Autodesk Inventor part; units mm, degrees
ref_plane "YZ Plane" through (0, 0, 0) normal (1, 0, 0) x (0, 1, 0)
ref_plane "XZ Plane" through (0, 0, 0) normal (0, 1, 0) x (-1, 0, 0)
ref_plane "XY Plane" through (0, 0, 0) normal (0, 0, 1) x (1, 0, 0)
sketch "card+border" plane through (0, 0, 0) normal (0, 0, 1) x (1, 0, 0)
  line L0 (-59.3579, 68.5808) -> (-59.3579, 10.0008)
  line L1 (-59.3579, 10.0008) -> (14.2921, 10.0008)
  line L2 (14.2921, 10.0008) -> (14.2921, 68.5808)
  line L3 (14.2921, 68.5808) -> (-59.3579, 68.5808)
  circle A0 centre (11.6671, 65.9558) radius 1.575
  circle A1 centre (11.6671, 12.6258) radius 1.575
  circle A2 centre (-56.7329, 65.9558) radius 1.575
  circle A3 centre (-56.7329, 12.6258) radius 1.575
  line L4 (-61.3579, 70.5808) -> (-61.3579, 8.0008)
  line L5 (-61.3579, 8.0008) -> (16.2921, 8.0008)
  line L6 (16.2921, 8.0008) -> (16.2921, 70.5808)
  line L7 (16.2921, 70.5808) -> (-61.3579, 70.5808)
  line L8 (-58.3579, 67.5808) -> (13.2921, 67.5808)
  line L9 (13.2921, 67.5808) -> (13.2921, 11.0008)
  line L10 (13.2921, 11.0008) -> (-58.3579, 11.0008)
  line L11 (-58.3579, 11.0008) -> (-58.3579, 67.5808)
  circle A4 centre (-56.7329, 65.9558) radius 3
  circle A5 centre (11.6671, 65.9558) radius 3
  circle A6 centre (11.6671, 12.6258) radius 3
  circle A7 centre (-56.7329, 12.6258) radius 3
  point P0 (0, 0)
  point P1 (-54.2111, 67.5808)
  point P2 (9.1454, 67.5808)
  point P3 (13.2921, 63.434)
  point P4 (13.2921, 15.1475)
  point P5 (9.1454, 11.0008)
  point P6 (-54.2111, 11.0008)
  point P7 (-58.3579, 15.1475)
  point P8 (-58.3579, 63.434)
  dimension "d1" = 58.58
  dimension "d2" = 73.65
  dimension "d4" = 2.625
  dimension "d5" = 3.15
  dimension "d31" = 2.625
  dimension "d32" = 2.625
  dimension "d33" = 2.625
  dimension "d34" = 3.15
  dimension "d35" = 2
  dimension "d36" = 3
  dimension "d37" = 3
  dimension "d38" = 3
  dimension "d39" = 3
  dimension "d40" = 6
  dimension "d41" = 6
  dimension "d42" = 6
  dimension "d43" = 6
extrude "Middle wall" add sketch "card+border" along normal blind 2 contours L3 A4 L0 | A4 L3 L8 L11 L0 | L0 A4 | A4 L3 | A4 L11 A7 L0 | L3 A5 L8 A4 | A7 L11 L10 L1 L0 | L0 A7 | L11 L8 A4 | A5 L3 | L3 A5 L2 L9 L8 | A7 L1 L0 | A7 L10 L11 | L3 L2 A5 | L8 L9 A5 | L1 A7 | A5 L2 | A5 L2 A6 L9 | A7 L10 A6 L1 | A6 L2 L1 L10 L9 | L9 L10 A6 | L1 A6 | A6 L2 | A6 L2 L1 | L7 L6 L5 L4
fillet "Skruehull suport" radius 2 8 edges at (9.1454, 67.5808, 1) (13.2921, 63.434, 1) (-58.3579, 63.434, 1) (-54.2111, 67.5808, 1) (-54.2111, 11.0008, 1) (-58.3579, 15.1475, 1) (13.2921, 15.1475, 1) (9.1454, 11.0008, 1)
fillet "Kantutjevning" radius 5 4 edges at (16.2921, 70.5808, 1) (-61.3579, 70.5808, 1) (-61.3579, 8.0008, 1) (16.2921, 8.0008, 1)
properties part number "Trippeldekker_Midtre plate"
CAD build for the part. Positions are in the model's coordinates, mm. A direction names the side the tool comes from. Coordinates: 2 decimals unless noted, no trailing zeros. Write each loop counter-clockwise with the first axis right and the second up, starting at its lowest first coordinate (ties: lowest second). Pieces come first, ordered by that corner, then holes. Notation, with made-up numbers: M 22,10 L 54,10 A21 ccw 54,45 Z; hole C 88.5,-16.75 d9. An arc over 180 degrees is marked long. Return JSON: item names as keys, results as strings.
Item 1: Slice it at C-C, the plane z = 1.25. Write the cut outline in (x, y) (3 decimals).
Findings below:
{"outline": "M -61.358,13.001 A5 ccw -56.358,8.001 L 11.292,8.001 A5 ccw 16.292,13.001 L 16.292,65.581 A5 ccw 11.292,70.581 L -56.358,70.581 A5 ccw -61.358,65.581 Z; hole M -58.358,17.612 A2 ccw -56.508,15.617 A3 cw -53.741,12.851 A2 ccw -51.747,11.001 L 6.681,11.001 A2 ccw 8.676,12.851 A3 cw 11.442,15.617 A2 ccw 13.292,17.612 L 13.292,60.97 A2 ccw 11.442,62.964 A3 cw 8.676,65.731 A2 ccw 6.681,67.581 L -51.747,67.581 A2 ccw -53.741,65.731 A3 cw -56.508,62.964 A2 ccw -58.358,60.97 Z; hole C -56.733,12.626 d3.15; hole C -56.733,65.956 d3.15; hole C 11.667,12.626 d3.15; hole C 11.667,65.956 d3.15"}
Item 2: Slice it at B-B, the plane y = 60. Write the cut outline in (x, z).
Findings below:
{"outline": "M -61.36,0 L -58.36,0 L -58.36,2 L -61.36,2 Z; M 13.29,0 L 16.29,0 L 16.29,2 L 13.29,2 Z"}
Item 3: Drop a flat-ended pin along its axis: pin 1 Ø3.5 at (x, y) = (11.67, 12.63) entering from -Z. Give the stop position or say it passes through.
Findings below:
{"pin 1": "stops at z = 0"}
Item 4: Which spindle directions (+Z, -Z, +X, -X, +Y, -Y) get a long thin tool onto all of the face, cutting with end or side? Do faces 4 (the cylindrical face through (-57.81, 62.345, 1.014)), 5 (the cylindrical face through (14.866, 69.077, 1.014)). Say none if no direction does.
Findings below:
{"face 4": "+Z, -Z", "face 5": "+Z, -Z, +X, +Y"}
Item 5: Probe line 1 (X direction, y = 33.5, z = 1); line 2 (Y direction, x = -7, z = 1.65); line 3 (X direction, y = 66, z = 1.2). List the from-to ranges inside material, lowest first. Write a range as from..to.
Findings below:
{"line 1": "x = -61.36..-58.36, 13.29..16.29", "line 2": "y = 8..11, 67.58..70.58", "line 3": "x = -61.34..-58.31, -55.16..-53.7, 8.64..10.09, 13.24..16.27"}
Item 6: Two-plate mould, pull along Y, no slides. Class faces 1 (the cylindrical face through (-53.092, 67.061, 1.014)), 2 (the flat face through (-23, 9, 2)), 3 (the cylindrical face through (14.79, 9.43, 1.01)): +Y half, -Y half, draft (parallel to the pull), parting line (faces both ways), or undercut.
Findings below:
{"face 1": "undercut", "face 2": "draft", "face 3": "-Y half"}
Item 7: Slice it at A-A, the plane x = -1. Write the cut outline in (y, z).
Findings below:
{"outline": "M 8,0 L 11,0 L 11,2 L 8,2 Z; M 67.58,0 L 70.58,0 L 70.58,2 L 67.58,2 Z"}
